Here's how the part is built. I have some questions about the finished solid (model axes, mm). A direction names the side the tool comes from. Round coordinates to 2 decimals unless told otherwise and drop trailing zeros. Loops run counter-clockwise (first coordinate to the right, second up) from the corner with the lowest first, then second, coordinate; pieces in that order, holes last. Notation, with made-up numbers: (-21, 86.5) -> (-14, 86.5) arc R12 cw to (-14, 99.5) -> close; hole circle Ø1 at (11, 79). An arc over 180 degrees is marked (long way). Use one line per item in the form item = value. Start each with the question number.
Item 1: If we section it at A-A (x = -49.5): Write out the boundary of the cut face in (y, z).
Item 2: If we section it at D-D (x = -29): Write out the boundary of the cut face in (y, z).
Item 3: If I drill on L1, parallel to Y at x = 4, z = 1.2; L2, parallel to Y at x = -43.5, z = -21; L3, parallel to Z at x = -56, y = -53.5, over which ranges is the centre line in solid material (lowest first)? Write a range as [from, to].
Item 4: I'm going to push flat-ended pins straight in: pin 1 Ø5.5 at (x, z) = (0, -8) entering from +Y; pin 2 Ø3 at (y, z) = (-8, -19.5) entering from -X; pin 3 Ø12 at (y, z) = (-4.5, -3.5) entering from +X; pin 4 Ø1.2 at (x, z) = (-46, -21) entering from +Y. Where does each tip first touch, or does it pass through?
Item 5: Thinking about a two-plate mould opening in Y: for faces 6 (the face through (-17.4, -44.735, -20.986)), 7 (the face through (-23, -51, -24)), 8 (the face through (-2.614, -6.575, 1.972)), which applies, released by +Y, released by -Y, zero draft, split by the parting line, or undercut?
Item 6: For faces 1 (the face through (0, -10, -12)), 2 (the face through (-6.9, -24.75, -23.43)), 3 (the face through (-7.5, -15, -9)), 4 (the face through (6.93, -10.6, -11.86)), 5 (the face through (-15.238, -46.373, -20.74)), which set-ups out of +Z, -Z, +X, -X, +Y, -Y let a thin tool reach every point of the face, with its end or its side?
Item 7: If we section it at C-C (y = -29): Write out the boundary of the cut face in (x, z), then the cut area to 3 significant figures.
```python
from build123d import *

# Parameters (mm, degrees)
SKETCH_1_W          = 15
SKETCH_1_H          = 26
SKETCH_1_R          = 2.5
SKETCH_1_R_2        = 1.5
EXTRUDE_1_DEPTH     = 4
SKETCH_3_W          = 15
SKETCH_3_H          = 6
EXTRUDE_2_DEPTH     = 20
EXTRUDE_3_DEPTH     = 4
SKETCH_9_W          = 40
SKETCH_9_H          = 10
CUT_EXTRUDE_1_DEPTH = 1.5
SKETCH_10_R         = 1.5
CUT_EXTRUDE_2_DEPTH = 4
CUT_EXTRUDE_3_DEPTH = 1.5
SKETCH_12_R         = 1.5
CUT_EXTRUDE_4_DEPTH = 10
FILLET_1_R          = 2
FILLET_2_R          = 2
FILLET_3_R          = 1


with BuildPart() as part:
    # 草图1 → 凸台-拉伸1 (new body)
    with BuildSketch(Plane.XY):
        with Locations((0, -3)):
            Rectangle(SKETCH_1_W, SKETCH_1_H)
        Circle(SKETCH_1_R, mode=Mode.SUBTRACT)
        with Locations((4, 6)):
            Circle(SKETCH_1_R_2, mode=Mode.SUBTRACT)
        with Locations((-4, -6)):
            Circle(SKETCH_1_R_2, mode=Mode.SUBTRACT)
    extrude(amount=EXTRUDE_1_DEPTH)

    # 草图3 → 凸台-拉伸2 (add)
    with BuildSketch(Plane(origin=(0, 0, 0), x_dir=(-1, 0, 0), z_dir=(0, 0, -1))):
        with Locations((0, -13)):
            Rectangle(SKETCH_3_W, SKETCH_3_H)
    extrude(amount=EXTRUDE_2_DEPTH)

    # 草图8 → 凸台-拉伸3 (add)
    with BuildSketch(Plane(origin=(0, 0, -20), x_dir=(-1, 0, 0), z_dir=(0, 0, -1))):
        Polygon((-7.5, -16), (-7.5, -47.679491924), (22.5, -65), (77.5, -65), (77.5, -50), (26.519237886, -50), (7.5, -39.019237886), (7.5, -16), (7.5, -10), (-7.5, -10), align=None)
    extrude(amount=EXTRUDE_3_DEPTH)

    # 草图9 → 切除-拉伸1 (cut)
    with BuildSketch(Plane.XY.offset(-20)):
        with Locations((-54.5, -57.5)):
            Rectangle(SKETCH_9_W, SKETCH_9_H)
    extrude(amount=-CUT_EXTRUDE_1_DEPTH, mode=Mode.SUBTRACT)

    # 草图10 → 切除-拉伸2 (cut)
    with BuildSketch(Plane.XY.offset(-21.5)):
        with Locations((-69.5, -57.5)):
            Circle(SKETCH_10_R)
        with Locations((-59.5, -57.5)):
            Circle(SKETCH_10_R)
        with Locations((-49.5, -57.5)):
            Circle(SKETCH_10_R)
        with Locations((-39.5, -57.5)):
            Circle(SKETCH_10_R)
    extrude(amount=-CUT_EXTRUDE_2_DEPTH, mode=Mode.SUBTRACT)

    # 草图11 → 切除-拉伸3 (cut)
    with BuildSketch(Plane.XY.offset(-20)):
        Polygon((-6.698729811, -41.443375673), (-24.019237886, -51.443375673), (-19.019237886, -60.103629711), (-1.698729811, -50.103629711), align=None)
    extrude(amount=-CUT_EXTRUDE_3_DEPTH, mode=Mode.SUBTRACT)

    # 草图12 → 切除-拉伸4 (cut)
    with BuildSketch(Plane.XY.offset(-21.5)):
        with Locations((-17.189110868, -53.273502692)):
            Circle(SKETCH_12_R)
        with Locations((-8.52885683, -48.273502692)):
            Circle(SKETCH_12_R)
    extrude(amount=-CUT_EXTRUDE_4_DEPTH, mode=Mode.SUBTRACT)

    # 圆角1
    fillet_1_edges = [part.edges().sort_by_distance(p)[0] for p in [
        (7.5, 0, 0),
        (7.5, -10, -12),
        (0, -10, 0),
        (-7.5, -10, -12),
        (0, -16, -20),
        (-77.5, -65, -22),
        (-77.5, -50, -22),
        (-26.519237886, -50, -22),
        (-7.5, -39.019237886, -22),
        (0, -10, -24),
        (7.5, -28.839745962, -24),
        (-50, -65, -24),
        (-77.5, -57.5, -24),
        (-52.009618943, -50, -24),
        (-17.009618943, -44.509618943, -24),
        (-7.5, -24.509618943, -24),
        (-7.5, 0, 0),
    ]]
    fillet(fillet_1_edges, radius=FILLET_1_R - 0.0001)  # a hair under: the kernel refuses the full size

    # 圆角2
    fillet_2_edges = [part.edges().sort_by_distance(p)[0] for p in [
        (0, -16, 4),
    ]]
    fillet(fillet_2_edges, radius=FILLET_2_R)

    # 圆角3
    fillet_3_edges = [part.edges().sort_by_distance(p)[0] for p in [
        (0, 10, 0),
        (-6.914242852, 10, 0.585757148),
        (6.914242852, 10, 0.585757148),
        (-7.5, 10, 2.99995),
        (7.5, 10, 2.99995),
    ]]
    fillet(fillet_3_edges, radius=FILLET_3_R)


solid = part.part
```
Values found:
q1.outline = (-65, -22) arc R2 ccw to (-63, -24) -> (-59, -24) -> (-59, -21.5) -> (-62.5, -21.5) -> (-62.5, -20) -> (-65, -20) -> close; (-56, -24) -> (-52, -24) arc R2 ccw to (-50, -22) -> (-50, -20) -> (-52.5, -20) -> (-52.5, -21.5) -> (-56, -21.5) -> close
q2.outline = (-65, -22) arc R2 ccw to (-63, -24) -> (-52, -24) arc R2 ccw to (-50, -22) -> (-50, -20) -> (-65, -20) -> close
q3.L1 = [-16, 4.5], [7.5, 10]
q3.L2 = [-65, -62.5], [-52.5, -50]
q3.L3 = [-24, -21.5]
q4.pin_1 = -10
q4.pin_2 = through
q4.pin_3 = 7.5
q4.pin_4 = -50
q5.face_6 = released by +Y
q5.face_7 = zero draft
q5.face_8 = undercut
q6.face_1 = -Z, +X, -X, +Y
q6.face_2 = -Z, -X, +Y
q6.face_3 = +Z, -Z, -X, +Y
q6.face_4 = -Z, +X, +Y
q6.face_5 = +Z
q7.outline = (-7.5, -22) arc R2 ccw to (-5.5, -24) -> (5.5, -24) arc R2 ccw to (7.5, -22) -> (7.5, -20) -> (-7.5, -20) -> close
q7.area = 58.3 mm2
